Work out the finished part from the listing and answer in its coordinate system (mm). Face numbers are marked on the shaded views. Round coordinates to 2 decimals unless told otherwise and drop trailing zeros. Order: outer loops, then holes, each group sorted by start corner. A loop starts at its lowest first (then second) coordinate and runs counter-clockwise, first axis right, second up. Notation, with made-up numbers: (32.25, 49) -> (75.25, 49) arc R33 cw to (75.25, 80) -> close; hole circle Ø8 at (-19.75, 40). An arc over 180 degrees is marked (long way). Use a Markdown table: item, result. Add a question column.
Item 1: A cutting plane is placed at C-C, the plane z = 4.25. Determine the outline of the cut face in (x, y).
Item 2: Flat-ended cylindrical pins translate along their axes: P1, Ø12, axis at y = -37.5, z = 22.5, coming from the +X side; P2, Ø12, axis at y = -33, z = 5, coming from the +X side; P3, Ø5, axis at x = 6.5, z = 9.5, coming from the -Y side. Find the tip coordinate at first contact, or state that the pin passes through.
Item 3: A cutting plane is placed at A-A, the plane z = 9. Determine the outline of the cut face in (x, y) (3 decimals), plus the area to 3 significant figures.
Item 4: Find the intervals of material crossed by L1, parallel to Y at x = 0, z = 11 (3 decimals); L2, parallel to Y at x = -18.5, z = 6; L3, parallel to X at y = -18, z = 3.25, in increasing order. Write a range as [from, to].
Item 5: For a pull along Y with two mould halves and no side action, classify the marked faces 1, 2 and 3 as +Y half, -Y half, draft (parallel to the pull), parting line (faces both ways), or undercut.
Item 6: A cutting plane is placed at B-B, the plane y = 0. Determine the outline of the cut face in (x, z) (3 decimals), plus the area to 3 significant figures.
from build123d import *

# Parameters (mm, degrees)
F0_R     = 22.225
F1_DEPTH = 25.4
F2_R     = 6.35
F3_R     = 6.35


# Not quite as in the source:
# - a feature names something its author has since deleted; it is built from what else it names


with BuildPart() as f1:
    # F0 (on Top) → F1 (new body)
    with BuildSketch(Plane.XY):
        Polygon((0, -50.8), (43.9940905122, -25.4), (43.9940905122, 25.4), (0, 50.8), (-43.9940905122, 25.4), (-43.9940905122, -25.4), align=None)
        Circle(F0_R, mode=Mode.SUBTRACT)
    extrude(amount=F1_DEPTH)

    # F2
    f2_edges = [f1.edges().sort_by_distance(p)[0] for p in [
        (-43.994091, -25.4, 12.7),
        (-43.994091, 25.4, 12.7),
        (0, -50.8, 12.7),
        (43.994091, -25.4, 12.7),
        (43.994091, 25.4, 12.7),
        (0, 50.8, 12.7),
    ]]
    fillet(f2_edges, radius=F2_R)

    # F3
    f3_edges = [f1.edges().sort_by_distance(p)[0] for p in [
        (-21.997045, -38.1, 25.4),
        (-21.997045, -38.1, 0),
        (-22.225, 0, 25.4),
        (-22.225, 0, 0),
    ]]
    fillet(f3_edges, radius=F3_R)


solid = f1.part
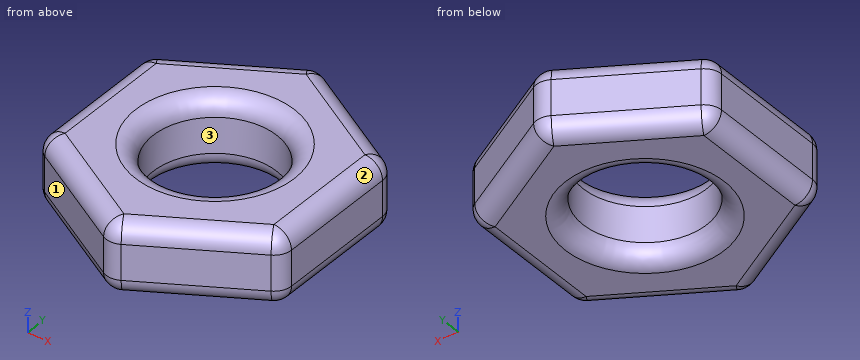
Reported:
| question | item | result |
|---|---|---|
| 1 | outline | (-43.64, -21.73) arc R5.99 ccw to (-40.64, -26.92) -> (-3, -48.66) arc R5.99 ccw to (3, -48.66) -> (40.64, -26.92) arc R5.99 ccw to (43.64, -21.73) -> (43.64, 21.73) arc R5.99 ccw to (40.64, 26.92) -> (3, 48.66) arc R5.99 ccw to (-3, 48.66) -> (-40.64, 26.92) arc R5.99 ccw to (-43.64, 21.73) -> close; hole circle Ø45.16 at (0, 0) |
| 2 | P1 | x = 32.51 |
| 2 | P2 | x = 41.07 |
| 2 | P3 | y = -48.49 |
| 3 | outline | (-43.994, -21.734) arc R6.35 ccw to (-40.819, -27.233) -> (-3.175, -48.967) arc R6.35 ccw to (3.175, -48.967) -> (40.819, -27.233) arc R6.35 ccw to (43.994, -21.734) -> (43.994, 21.734) arc R6.35 ccw to (40.819, 27.233) -> (3.175, 48.967) arc R6.35 ccw to (-3.175, 48.967) -> (-40.819, 27.233) arc R6.35 ccw to (-43.994, 21.734) -> close; hole circle Ø44.45 at (0, 0) |
| 3 | area | 5,140 mm² |
| 4 | L1 | [-49.818, -22.225], [22.225, 49.818] |
| 4 | L2 | [-40.11, -12.33], [12.33, 40.11] |
| 4 | L3 | [-43.19, -14.37], [14.37, 43.19] |
| 5 | face 1 | -Y half |
| 5 | face 2 | draft |
| 5 | face 3 | undercut |
| 6 | outline | (-43.994, 6.35) arc R6.35 ccw to (-37.644, 0) -> (-28.575, 0) arc R6.35 ccw to (-22.225, 6.35) -> (-22.225, 19.05) arc R6.35 ccw to (-28.575, 25.4) -> (-37.644, 25.4) arc R6.35 ccw to (-43.994, 19.05) -> close; (22.225, 6.35) arc R6.35 ccw to (28.575, 0) -> (37.644, 0) arc R6.35 ccw to (43.994, 6.35) -> (43.994, 19.05) arc R6.35 ccw to (37.644, 25.4) -> (28.575, 25.4) arc R6.35 ccw to (22.225, 19.05) -> close |
| 6 | area | 1,040 mm² |
